```python
from build123d import *

# Parameters (mm, degrees)
F1_DEPTH = 20


with BuildPart() as f1:
    # F0 (on Front) → F1 (new body)
    with BuildSketch(Plane.XZ):
        with BuildLine():
            Line((0, -12), (0, 0))
            Line((0, 0), (-200, 0))
            ThreePointArc((-200, 0), (-220, 20), (-200, 40))
            Line((-200, 40), (-180, 40))
            Line((-180, 40), (-180, 52))
            Line((-180, 52), (-200, 52))
            ThreePointArc((-200, 52), (-232, 20), (-200, -12))
            Line((-200, -12), (0, -12))
        make_face()
    extrude(amount=-F1_DEPTH)


solid = f1.part
```
Verification items for the finished model (mm, model axes). A direction names the side the tool comes from. Give positions to 0.01 mm unless a question says otherwise; leave off trailing zeros. Order: outer loops, then holes, each group sorted by start corner. A loop starts at its lowest first (then second) coordinate and runs counter-clockwise, first axis right, second up. Notation, with made-up numbers: M 38.5,81.5 L 52.5,81.5 A26 ccw 52.5,108.5 Z; hole C 67.25,78.25 d1. An arc over 180 degrees is marked long. Answer in a Markdown table with one row per item. Add a question column.
Item 1: Section check C-C, the plane z = 20. Enter the section's corners in (x, y), and give its area (3 significant figures).
Item 2: Tool access check on faces 4 (the flat face through (0, 10, -6)), 5 (the flat face through (-180, 10, 46)). Record the directions out of +Z, -Z, +X, -X, +Y, -Y that give a thin tool (end or side, any length) a straight path to the whole face; none if there is none.
Item 3: Section check B-B, the plane x = -51.5. Enter the section's corners in (y, z).
Item 4: Scan lines: probe 1 along Z at (x, y) = (-192, 4.75); probe 2 along Z at (x, y) = (-148, 3.5); probe 3 along X at (y, z) = (4.75, -5). Record each from-to range of solid material in increasing order. Write a range as from..to.
Item 5: Mould release check, pull along Z, two halves, no side actions. Record for faces 1 (the flat face through (-101, 10, -12)), 2 (the flat face through (-190, 10, 40)), 3 (the flat face through (-190, 10, 52)): released by +Z, released by -Z, zero draft, split by the parting line, or undercut.
Item 6: Section check A-A, the plane y = 11. Enter the section's corners in (x, z), and give its area (3 significant figures).
Item 7: Gauge pin test, flat ends, axial feed: pin 1 (1 mm diameter, centred on x = -111.5, y = 13, fed in from +Z); pin 2 (3.5 mm diameter, centred on y = 6.5, z = 44, fed in from +X); pin 3 (1.5 mm diameter, centred on y = 14, z = 19, fed in from -X). Record the tip position at first contact, or that the pin passes through.
Filled sheet:
| question | item | result |
|---|---|---|
| 1 | outline | M -232,0 L -220,0 L -220,20 L -232,20 Z |
| 1 | area | 240 mm^2 |
| 2 | face 4 | +Z, -Z, +X, +Y, -Y |
| 2 | face 5 | +Z, +X, +Y, -Y |
| 3 | outline | M 0,-12 L 20,-12 L 20,0 L 0,0 Z |
| 4 | probe 1 | z = -12..0, 40..52 |
| 4 | probe 2 | z = -12..0 |
| 4 | probe 3 | x = -219.97..0 |
| 5 | face 1 | released by -Z |
| 5 | face 2 | undercut |
| 5 | face 3 | released by +Z |
| 6 | outline | M -200,-12 L 0,-12 L 0,0 L -200,0 A20 cw -200,40 L -180,40 L -180,52 L -200,52 A32 ccw Z |
| 6 | area | 3,620 mm^2 |
| 7 | pin 1 | stops at z = 0 |
| 7 | pin 2 | stops at x = -180 |
| 7 | pin 3 | stops at x = -232 |
